Verification items for the finished model (mm, model axes). A direction names the side the tool comes from. Coordinates: 2 decimals unless noted, no trailing zeros. Loops run counter-clockwise (first coordinate to the right, second up) from the corner with the lowest first, then second, coordinate; pieces in that order, holes last. Notation, with made-up numbers: M 29.25,86.25 L 63.25,86.25 A26 cw 63.25,113.25 Z; hole C -28.5,73 d4. An arc over 180 degrees is marked long. Write item = value, one per line. Start each with the question number.
```python
from build123d import *

# Parameters (mm, degrees)
F0_W     = 45
F0_H     = 75
F0_R     = 1.27
F1_DEPTH = 2
F2_DEPTH = 10


with BuildPart() as f1:
    # F0 (on Top) → F1 (new body)
    with BuildSketch(Plane.XY):
        Rectangle(F0_W, F0_H)
        with Locations((-20.230002, -32.42)):
            Circle(F0_R, mode=Mode.SUBTRACT)
        with Locations((-12.7, -31.15)):
            Circle(F0_R, mode=Mode.SUBTRACT)
        with Locations((12.7, -31.15)):
            Circle(F0_R, mode=Mode.SUBTRACT)
        with Locations((20.230002, -32.42)):
            Circle(F0_R, mode=Mode.SUBTRACT)
        with Locations((-20.230002, 35.23)):
            Circle(F0_R, mode=Mode.SUBTRACT)
        with Locations((-12.7, 31.15)):
            Circle(F0_R, mode=Mode.SUBTRACT)
        with Locations((12.7, 31.15)):
            Circle(F0_R, mode=Mode.SUBTRACT)
        with Locations((20.23, 35.230002)):
            Circle(F0_R, mode=Mode.SUBTRACT)
        with Locations((-20.230002, -32.42)):
            Circle(F0_R)
        with Locations((20.230002, -32.42)):
            Circle(F0_R)
        with Locations((20.23, 35.230002)):
            Circle(F0_R)
        with Locations((-20.230002, 35.23)):
            Circle(F0_R)
    extrude(amount=F1_DEPTH)

    # F0 (on Top) → F2 (join)
    with BuildSketch(Plane.XY):
        with Locations((-20.230002, 35.23)):
            Circle(F0_R)
        with Locations((20.230002, -32.42)):
            Circle(F0_R)
        with Locations((-20.230002, -32.42)):
            Circle(F0_R)
        with Locations((20.23, 35.230002)):
            Circle(F0_R)
    extrude(amount=F2_DEPTH)


solid = f1.part
```
Q1. Sectioned sample at D-D on y = 5.5. Record the cut outline in (x, z).
Q2. Sectioned sample at C-C on x = 20.23. Record the cut outline in (y, z), plus the area to 3 significant figures.
Q3. Scan lines: L1, parallel to Y at x = 12.7, z = 0.8; L2, parallel to Z at x = -14, y = -1. Record each from-to range of solid material in increasing order. Write a range as [from, to].
Q4. Sectioned sample at B-B on z = 7.25. Record the cut outline in (x, y).
Q5. Sectioned sample at A-A on x = -12.7. Record the cut outline in (y, z).
Q6. Set-up check for faces 1 (the face through (0, 1, 0)), 2 (the face through (19.22, 34.46, 5.94)): record each of +Z, -Z, +X, -X, +Y, -Y from which the full face is reachable in a straight line by a thin tool's end or side.
Q7. Mould release check, pull along X, two halves, no side actions. Record for faces 3 (the face through (-22.5, -1, 1)), 4 (the face through (-20, -32, 10)), 5 (the face through (-20.51, -33.66, 5.94)), 6 (the face through (22.5, -1, 1)): +X half, -X half, draft (parallel to the pull), parting line (faces both ways), or undercut.
Q8. Gauge pin test, flat end, axial feed: pin 1 (5 mm diameter, centred on x = 11, y = -0.5, fed in from +Z). Record the tip position at first contact, or that the pin passes through.
Solutions:
q1.outline = M -22.5,0 L 22.5,0 L 22.5,2 L -22.5,2 Z
q2.outline = M -37.5,0 L 37.5,0 L 37.5,2 L 36.5,2 L 36.5,10 L 33.96,10 L 33.96,2 L -31.15,2 L -31.15,10 L -33.69,10 L -33.69,2 L -37.5,2 Z
q2.area = 191 mm²
q3.L1 = [-37.5, -32.42], [-29.88, 29.88], [32.42, 37.5]
q3.L2 = [0, 2]
q4.outline = C -20.23,-32.42 d2.54; C -20.23,35.23 d2.54; C 20.23,-32.42 d2.54; C 20.23,35.23 d2.54
q5.outline = M -37.5,0 L -32.42,0 L -32.42,2 L -37.5,2 Z; M -29.88,0 L 29.88,0 L 29.88,2 L -29.88,2 Z; M 32.42,0 L 37.5,0 L 37.5,2 L 32.42,2 Z
q6.face_1 = -Z, +X, -X, +Y, -Y
q6.face_2 = +Z
q7.face_3 = -X half
q7.face_4 = draft
q7.face_5 = undercut
q7.face_6 = +X half
q8.pin_1 = 2
